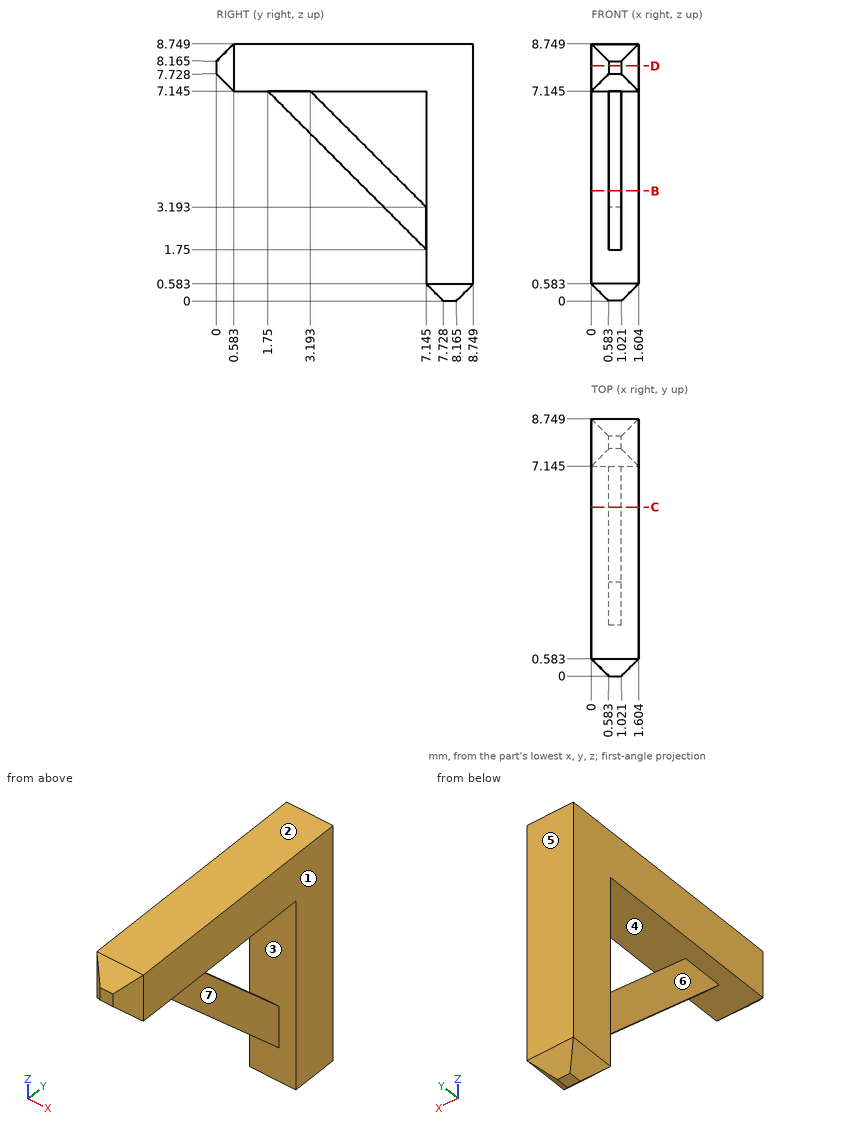
Print and shaded views of the part. All mm, measured from the part's lowest x, y and z. A direction names the side the tool comes from. Give positions to 0.01 mm unless a question says otherwise; leave off trailing zeros. Order: outer loops, then holes, each group sorted by start corner. A loop starts at its lowest first (then second) coordinate and runs counter-clockwise, first axis right, second up. Notation, with made-up numbers: (-12.5, 12.25) - (29.5, 12.25) arc R29 ccw to (29.5, 49.25) - close; hole circle Ø10 at (78, -27). An arc over 180 degrees is marked (long way). One line per item, written item: value.
Item 1: Pin check, flat tips, straight feed: pin 1 Ø0.5 at (x, y) = (1, 5.5) entering from -Z (1 decimal); pin 2 Ø1.6 at (y, z) = (4, 5) entering from -X. Stop position of each tip, or through.
Response values:
pin 1: z = 3.1
pin 2: x = 0.58
Item 2: Wall check: line 1 (Z direction, x = 1.3, y = 4.5) (1 decimal); line 2 (Z direction, x = 0.95, y = 7.5). Give the ranges that are in metal, low to high.
Response values:
line 1: 7.1 to 8.7
line 2: 0.23 to 8.75
Item 3: Slice it at B-B (z = 3.75). List the corners of the cut face in (x, y) (1 decimal).
Response values:
outline: (0, 7.1) - (1.6, 7.1) - (1.6, 8.7) - (0, 8.7) - close; (0.6, 5.1) - (1, 5.1) - (1, 6.6) - (0.6, 6.6) - close
Item 4: Slice it at C-C (y = 5.75). List the corners of the cut face in (x, z) (1 decimal).
Response values:
outline: (0, 7.1) - (1.6, 7.1) - (1.6, 8.7) - (0, 8.7) - close; (0.6, 3.1) - (1, 3.1) - (1, 4.6) - (0.6, 4.6) - close
Item 5: Two-plate mould, pull along Z, no slides. Class the marked faces 1, 2, 3 and 4: released by +Z, released by -Z, zero draft, split by the parting line, or undercut.
Response values:
face 1: zero draft
face 2: released by +Z
face 3: undercut
face 4: undercut
Item 6: Slice it at D-D (z = 8). List the corners of the cut face in (x, y).
Response values:
outline: (0, 0.58) - (0.58, 0) - (1.02, 0) - (1.6, 0.58) - (1.6, 8.75) - (0, 8.75) - close
Item 7: Tool access for the marked faces 5, 6 and 7: list every direction of +Z, -Z, +X, -X, +Y, -Y with a clear straight run to the whole face (end or side of a thin tool).
Response values:
face 5: +Z, -Z, +X, -X, +Y
face 6: -Z, -X, -Y
face 7: -Z, +X, -Y
